Autodesk Inventor part; units mm, degrees
ref_plane "YZ Plane" through (0, 0, 0) normal (1, 0, 0) x (0, 1, 0)
ref_plane "XZ Plane" through (0, 0, 0) normal (0, 1, 0) x (-1, 0, 0)
ref_plane "XY Plane" through (0, 0, 0) normal (0, 0, 1) x (1, 0, 0)
sketch "Sketch1" plane through (0, 0, 0) normal (0, 0, 1) x (1, 0, 0)
  line L0 (38.3225, 4.6263) -> (24.416, 4.6263)
  line L1 (38.3225, 4.6263) -> (38.3225, 37.1129)
  line L2 (38.3225, 37.1129) -> (24.416, 37.1129)
  line L3 (24.416, 37.1129) -> (24.416, 4.6263)
  line L4 (9.8554, 1.6101) -> (9.8554, 40.1292)
  line L5 (9.8554, 40.1292) -> (19.6852, 40.1292)
  line L6 (19.6852, 40.1292) -> (19.6852, 1.6101)
  line L7 (19.6852, 1.6101) -> (9.8554, 1.6101)
  line L8 (31.3692, 4.6263) -> (31.3692, 37.1129)
  line L9 (52.883, 1.6101) -> (52.883, 40.1292)
  line L10 (52.883, 40.1292) -> (43.0532, 40.1292)
  line L11 (43.0532, 40.1292) -> (43.0532, 1.6101)
  line L12 (43.0532, 1.6101) -> (52.883, 1.6101)
  point P0 (0, 0)
  point P1 (9.8554, 20.8696)
  point P2 (52.883, 20.8696)
  dimension "d0" = 13.9065
  dimension "d1" = 32.4866
  dimension "d2" = 38.5191
  dimension "d3" = 16.2433
  dimension "d5" = 9.8298
  dimension "d31" = 43.0276
  dimension "d59" = 38.5191
extrude "Extrusion6" add sketch "Sketch1" along normal blind 3.048 contours L4 L5 L6 L7 | L12 L11 L10 L9
extrude "Extrusion7" add sketch "Sketch1" along normal blind 10.287 contours L0 L8 L2 L1 | L0 L3 L2 L8
sketch "Sketch6" plane through (24.416, 37.1129, 0) normal (0, 1, 0) x (1, 0, 0)
  line L0 (13.9065, 0) -> (0, 0)
  line L1 (0, 0) -> (0, -10.287)
  line L2 (13.9065, -10.287) -> (0, -10.287)
  line L3 (13.9065, 0) -> (13.9065, -10.287)
  line L4 (13.9065, -7.239) -> (0, -7.239)
  point P0 (-24.416, 0)
  dimension "d36" = 3.048
extrude "Extrusion8" cut sketch "Sketch6" against normal blind 50.8 contours L3 L4 L1 L0
sketch "Sketch7" plane through (24.416, 37.1129, 10.287) normal (0, 1, 0) x (1, 0, 0)
  line L0 (28.4671, 7.239) -> (18.6373, 7.239)
  line L1 (0, 0) -> (13.9065, 0)
  line L2 (20.4193, 12.3132) -> (10.4121, 0.6025)
  line L3 (23.3323, 11.0303) -> (13.9065, 0)
  line L4 (13.9065, 3.048) -> (13.9065, 0)
  line L5 (13.9065, 0) -> (10.4121, 0)
  line L6 (10.4121, 0.6025) -> (10.4121, 0)
  line L7 (28.4671, 10.287) -> (18.6373, 10.287)
  line L8 (18.6373, 10.287) -> (18.6373, 7.239)
  line L9 (28.4671, 7.239) -> (18.6373, 7.239)
  line L10 (28.4671, 10.287) -> (28.4671, 7.239)
  line L11 (13.9065, 3.048) -> (0, 3.048)
  line L12 (0, 3.048) -> (0, 0)
  line L13 (13.9065, 0) -> (0, 0)
  line L14 (13.9065, 3.048) -> (13.9065, 0)
  line L15 (6.9533, 0) -> (6.9533, 10.1633)
  line L16 (-14.5606, 7.239) -> (-4.7307, 7.239)
  line L17 (-6.5128, 12.3132) -> (3.4944, 0.6025)
  line L18 (-9.4258, 11.0303) -> (0, 0)
  line L19 (0, 0) -> (3.4944, 0)
  line L20 (3.4944, 0.6025) -> (3.4944, 0)
  line L21 (-14.5606, 10.287) -> (-4.7307, 10.287)
  point P0 (-24.416, 10.287)
  point P1 (1.4047, 3.048)
  point P2 (-4.7813, 10.287)
  point P3 (-8.7906, 10.287)
  point P4 (12.5018, 3.048)
  point P5 (20.0925, 7.239)
  point P6 (18.6373, 10.2278)
  dimension "d39" = 3.048
  dimension "d40" = 0
  dimension "d41" = 0
extrude "Extrusion9" add sketch "Sketch7" against normal blind 32.4866 contours L3 L4 L11 L2 L8 L0 | L11 L12 L18 L21 L17
sketch "Sketch8" plane through (0, 0, 3.048) normal (0, 0, 1) x (1, 0, 0)
  circle A0 centre (14.6052, 7.9601) radius 3.175
  line L0 (9.8554, 1.6101) -> (19.6852, 1.6101)
  circle A1 centre (14.6052, 33.7792) radius 3.175
  line L1 (19.6852, 40.1292) -> (9.8554, 40.1292)
  line L2 (38.3225, 37.1129) -> (24.416, 37.1129)
  line L3 (24.416, 37.1129) -> (24.416, 4.6263)
  line L4 (24.416, 4.6263) -> (38.3225, 4.6263)
  line L5 (38.3225, 4.6263) -> (38.3225, 37.1129)
  line L6 (38.3225, 37.1129) -> (24.416, 37.1129)
  line L7 (31.3692, 37.1129) -> (31.3692, 17.7925)
  line L8 (19.6852, 1.6101) -> (19.6852, 40.1292)
  line L9 (19.6852, 1.6101) -> (19.6852, 4.6263)
  circle A2 centre (48.1332, 7.9601) radius 3.175
  circle A3 centre (48.1332, 33.7792) radius 3.175
  point P0 (0, 0)
  point P1 (19.6852, 37.1129)
  point P2 (19.6852, 38.6211)
  dimension "d44" = 6.35
  dimension "d45" = 6.35
  dimension "d46" = 6.35
  dimension "d47" = 6.35
  dimension "d55" = 5.08
  dimension "d56" = 5.08
fillet "Fillet4" radius 1.27 12 edges at (9.8554, 40.1292, 1.524) (19.6852, 40.1292, 1.524) (19.6852, 37.1129, 1.5536) (43.0532, 37.1129, 1.5536) (43.0532, 40.1292, 1.524) (52.883, 40.1292, 1.524) (52.883, 1.6101, 1.524) (43.0532, 1.6101, 1.524) (9.8554, 1.6101, 1.524) (19.6852, 1.6101, 1.524) (19.6852, 4.6263, 1.5536) (43.0532, 4.6263, 1.5536)
fillet "Fillet5" radius 6.35 2 edges at (24.416, 20.8696, 10.287) (38.3225, 20.8696, 10.287)
fillet "Fillet6" radius 1.27 1 edges at (18.23, 20.8696, 3.048)
fillet "Fillet7" radius 1.27 1 edges at (44.5085, 20.8696, 3.048)
fillet "Fillet8" radius 1.27 2 edges at (25.8207, 20.8696, 7.239) (36.9178, 20.8696, 7.239)
extrude "Extrusion11" cut sketch "Sketch8" against normal blind 50.8 contours A0 | A1 | A2 | A3
properties part number "Wheel Bracket"
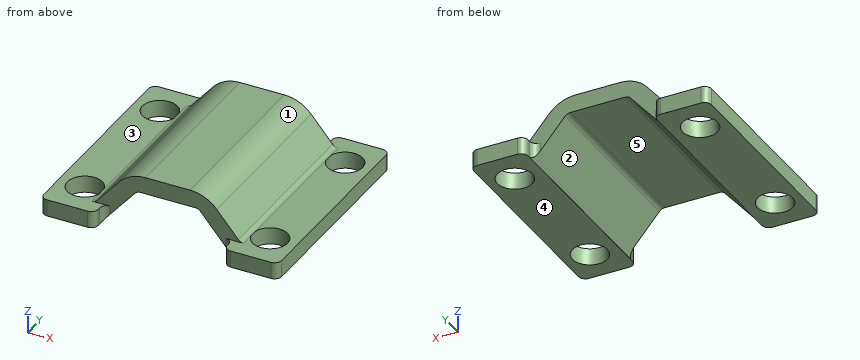
Design review of the part built by this model. Coordinates are the model's own, in mm. Face numbers are marked on the shaded views. A direction names the side the tool comes from. Coordinates: 2 decimals unless noted, no trailing zeros. Order: outer loops, then holes, each group sorted by start corner. A loop starts at its lowest first (then second) coordinate and runs counter-clockwise, first axis right, second up. Notation, with made-up numbers: (-21, -2.5) -> (25, -2.5) arc R27 ccw to (25, 30.5) -> close; hole circle Ø6 at (-8, -25.5). An arc over 180 degrees is marked (long way). Use one line per item in the form item = value. Start each with the question number.
(1) Add section A-A on x = 49.5. State the section outline as (y, z) points, plus the area to 3 significant figures.
(2) For the marked faces 4 and 5, list the 3-axis set-ups (+Z, -Z, +X, -X, +Y, -Y) from which the entire face can be reached by the end or side of a thin tool; tool diameter is ignored.
(3) Add section D-D on z = 4.25. State the section outline as (x, y) points.
(4) Add section C-C on y = 5.5. State the section outline as (x, z) points.
(5) The part is to be moulded in two halves that separate along X. For the marked faces 1, 2 and 3, say which applies: +X half, -X half, draft (parallel to the pull), parting line (faces both ways), or undercut.
(6) For probe 1 along X at (y, z) = (32, 2); probe 2 along Y at (x, z) = (13, 2.75); probe 3 along Y at (x, z) = (28, 7.5), list the stretches that pass through material, from the lowest coordinate up.
(7) Insertion check: pin 1 (4.5 mm diameter, centred on x = 32, z = 6, fed in from -Y); pin 2 (5.5 mm diameter, centred on x = 13.5, y = 29, fed in from +Z); pin 3 (4.5 mm diameter, centred on x = 29.5, z = 7.5, fed in from +Y); pin 4 (5 mm diameter, centred on x = 14.61, y = 7.96, fed in from -Z). Each pin has a flat end and moves straight along its axis. Give the tip position at first contact, or say it passes through.
(8) Add section B-B on z = 1. State the section outline as (x, y) points (3 decimals).
Answer block:
q1.outline = (1.61, 0) -> (5.09, 0) -> (5.09, 3.05) -> (1.61, 3.05) -> close; (10.83, 0) -> (30.91, 0) -> (30.91, 3.05) -> (10.83, 3.05) -> close; (36.64, 0) -> (40.13, 0) -> (40.13, 3.05) -> (36.64, 3.05) -> close
q1.area = 82.5 mm²
q2.face_4 = -Z, +X, -X, +Y, -Y
q2.face_5 = -Z, +Y, -Y
q3.outline = (19.26, 4.63) -> (23.27, 4.63) -> (23.27, 37.11) -> (19.26, 37.11) -> close; (39.47, 4.63) -> (43.48, 4.63) -> (43.48, 37.11) -> (39.47, 37.11) -> close
q4.outline = (9.86, 0) -> (12.6, 0) -> (12.6, 3.05) -> (9.86, 3.05) -> close; (16.61, 0) -> (19.69, 0) -> (19.69, 0.06) -> (25.44, 6.79) arc R1.27 cw to (26.41, 7.24) -> (36.33, 7.24) arc R1.27 cw to (37.3, 6.79) -> (43.05, 0.06) -> (43.05, 0) -> (46.13, 0) -> (46.13, 3.05) -> (45.09, 3.05) arc R1.27 cw to (44.13, 3.49) -> (40.22, 8.06) arc R6.35 ccw to (35.4, 10.29) -> (27.34, 10.29) arc R6.35 ccw to (22.51, 8.06) -> (18.61, 3.49) arc R1.27 cw to (17.64, 3.05) -> (16.61, 3.05) -> close; (50.14, 0) -> (52.88, 0) -> (52.88, 3.05) -> (50.14, 3.05) -> close
q5.face_1 = +X half
q5.face_2 = undercut
q5.face_3 = draft
q6.probe_1 = 9.86 to 11.98, 17.23 to 21.34, 41.39 to 45.5, 50.76 to 52.88
q6.probe_2 = 1.61 to 5.22, 10.7 to 31.04, 36.52 to 40.13
q6.probe_3 = 4.63 to 37.11
q7.pin_1 = 4.63
q7.pin_2 = 3.05
q7.pin_3 = 37.11
q7.pin_4 = through
q8.outline = (9.855, 2.88) arc R1.27 ccw to (11.125, 1.61) -> (18.415, 1.61) arc R1.27 ccw to (19.685, 2.88) -> (19.685, 3.356) arc R1.27 cw to (20.489, 4.538) -> (20.489, 37.201) arc R1.27 cw to (19.685, 38.383) -> (19.685, 38.859) arc R1.27 ccw to (18.415, 40.129) -> (11.125, 40.129) arc R1.27 ccw to (9.855, 38.859) -> close; (42.249, 4.538) arc R1.27 cw to (43.053, 3.356) -> (43.053, 2.88) arc R1.27 ccw to (44.323, 1.61) -> (51.613, 1.61) arc R1.27 ccw to (52.883, 2.88) -> (52.883, 38.859) arc R1.27 ccw to (51.613, 40.129) -> (44.323, 40.129) arc R1.27 ccw to (43.053, 38.859) -> (43.053, 38.383) arc R1.27 cw to (42.249, 37.202) -> close; hole circle Ø6.35 at (14.605, 7.96); hole circle Ø6.35 at (14.605, 33.779); hole circle Ø6.35 at (48.133, 7.96); hole circle Ø6.35 at (48.133, 33.779)
